Autodesk Inventor part; units mm, degrees
ref_plane "Plan de construction1" through (0, 10, 0) normal (0, 1, 0) x (-1, 0, 0)
ref_plane "YZ Plane" through (0, 0, 0) normal (1, 0, 0) x (0, 1, 0)
ref_plane "XY Plane" through (0, 0, 0) normal (0, 0, 1) x (1, 0, 0)
sketch "Esquisse1" plane through (0, 0, 0) normal (0, 0, 1) x (1, 0, 0)
  line L0 (0, 0) -> (0, 38)
  line L1 (0, 38) -> (30, 38)
  line L2 (30, 38) -> (30, 35.5)
  line L3 (30, 35.5) -> (0, 35.5)
  line L4 (0, 0) -> (0, 10)
  line L5 (0, 10) -> (18, 10)
  line L6 (18, 10) -> (18, 0)
  line L7 (18, 0) -> (0, 0)
  line L8 (-6, 0) -> (36, 0)
  dimension "d0" = 38
  dimension "d1" = 30
  dimension "d2" = 2.5
  dimension "d3" = 10
  dimension "d4" = 18
revolve "Révolution1" add sketch "Esquisse1" angle 360 about axis through (-10, 0, 0) along (1, 0, 0)
ref_plane "Plan de construction1" through (0, 10, 0) normal (0, 1, 0) x (-1, 0, 0)
sketch "Esquisse2" plane through (0, 10, 0) normal (0, 1, 0) x (-1, 0, 0)
  line L0 (0, 0) -> (0, 1)
  line L1 (0, 38) -> (0, -38)
  line L2 (0, 1) -> (-18, 1)
  line L3 (-18, 1) -> (-18, -1)
  line L4 (-18, -1) -> (0, -1)
  line L5 (0, 0) -> (0, -1)
  dimension "d7" = 1
  dimension "d8" = 18
  dimension "d9" = 2
  dimension "d10" = 90
extrude "Extrusion1" add sketch "Esquisse2" along normal up to surface
sketch "Esquisse3" plane through (30, 0, 0) normal (1, 0, 0) x (0, 0, -1)
  circle A0 centre (0, 0) radius 38
  circle A1 centre (0, 0) radius 38
  line L0 (0, 38) -> (0, 40)
  line L1 (0, 40) -> (0.5, 40)
  line L2 (0.5, 40) -> (0.5, 37.9967)
  line L3 (0, 40) -> (-0.5, 40)
  line L4 (-0.5, 40) -> (-0.5, 37.9967)
  dimension "d13" = 2
  dimension "d14" = 0.5
  dimension "d15" = 0.5
extrude "Extrusion2" add sketch "Esquisse3" against normal blind 30 contours A0 L0 L1 L2 | L4 L3 L0 A0
pattern_circular "Réseau circulaire1" count 10 over 360 about axis through (9, 0, 0) along (1, 0, 0) of "Extrusion1"
pattern_circular "Réseau circulaire2" count 40 over 360 about axis through (9, 0, 0) along (1, 0, 0) of "Extrusion2"
sketch "Esquisse4" plane through (0, 0, 0) normal (-1, 0, 0) x (0, 0, 1)
  circle A0 centre (0, 0) radius 2.85
  circle A1 centre (0, 0) radius 2.65
  line L0 (2.65, 0) -> (-2, 0)
  line L1 (-2, 0) -> (-2, 1.7385)
  line L2 (-2, 0) -> (-2, -1.7385)
  point P0 (-1.816, -1.3284)
  point P1 (-1.816, 1.3284)
  dimension "d24" = 5.7
  dimension "d25" = 5.3
  dimension "d26" = 4.65
extrude "Extrusion3" cut sketch "Esquisse4" against normal blind 25 contours L0 L1 A1 | A1 L2 L0
sketch "Esquisse7" plane through (0, 0, 0) normal (-1, 0, 0) x (0, 0, 1)
  circle A0 centre (0, 0) radius 2.55
  dimension "d30" = 5.1
extrude "Extrusion4" cut sketch "Esquisse7" against normal blind 7
sketch "Esquisse8" plane through (0, 0, 0) normal (-1, 0, 0) x (0, 0, 1)
  arc A0 (-2, 1.5819) -> (-2, -1.5819) centre (0, 0) ccw
  circle A1 centre (0, 0) radius 35.5
  line L0 (-2, 1.5819) -> (-2, -1.5819)
  arc A2 (-2, 1.5819) -> (-2, -1.5819) centre (0, 0) ccw
extrude "Extrusion5" cut sketch "Esquisse8" against normal blind 4 contours L0 A0 | A1
sketch "Esquisse9" plane through (18, 0, 0) normal (1, 0, 0) x (0, 0, -1)
  arc A0 (2, -1.5819) -> (2, 1.5819) centre (0, 0) ccw
  circle A1 centre (0, 0) radius 7.0446
  circle A2 centre (0, 0) radius 44.6529
extrude "Extrusion6" cut sketch "Esquisse9" along normal through all both and the other way through all
properties part number "Roue test"
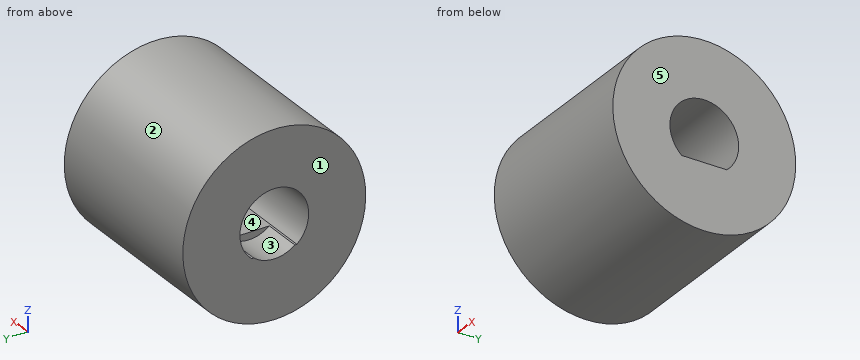
Could you check a few things on this model? Use its own coordinates, in mm. Face numbers are marked on the shaded views. A direction names the side the tool comes from. Give positions to 0.01 mm unless a question says otherwise; leave off trailing zeros. Write each loop counter-clockwise with the first axis right and the second up, starting at its lowest first coordinate (ties: lowest second). Pieces come first, ordered by that corner, then holes. Notation, with made-up numbers: (55.5, -33.75) -> (61.5, -33.75) arc R15 cw to (61.5, -8.75) -> close; hole circle Ø4 at (50, -19). An arc over 180 degrees is marked (long way). Write each question's results on one line, items separated by ' | '. Start each with the question number.
Q1. Suppose I cut it at A-A, the plane z = 0. List the corners of the cut face in (x, y) for me, and give its area (3 significant figures).
Q2. We'd pull the mould along Y, two halves only. Please class the marked faces 1, 2 and 3: +Y half, -Y half, draft (parallel to the pull), parting line (faces both ways), or undercut.
Q3. Which directions (+Z, -Z, +X, -X, +Y, -Y) give clear straight access to the entire face, cutting with the end or side of a thin tool? Please do the marked faces 4 and 5.
Q4. Suppose I cut it at D-D, the plane z = 2.25. List the corners of the cut face in (x, y) for me, and give its area (3 significant figures).
Q5. Suppose I cut it at C-C, the plane x = 8.5. List the corners of the cut face in (y, z) for me.
Q6. I'm going to push flat-ended pins straight in: pin 1 Ø4 at (x, y) = (14, 4.5) entering from +Z; pin 2 Ø3 at (x, z) = (15.5, 4) entering from -Y; pin 3 Ø2 at (x, y) = (8.5, -2) entering from +Z. Where does each tip first touch, or does it pass through?
Q7. I need wall thicknesses on probe 1 along Y at (x, z) = (10.5, 0); probe 2 along Z at (x, y) = (13.5, 1.75); probe 3 along Z at (x, y) = (8.25, 2). Which ranges of each line are inside material? Lowest first, please.
Q8. Suppose I cut it at B-B, the plane y = -0.5. List the corners of the cut face in (x, z) for me.
Outcome:
1) outline: (4, -7.04) -> (18, -7.04) -> (18, -2.65) -> (4, -2.65) -> close; (4, 2.65) -> (18, 2.65) -> (18, 7.04) -> (4, 7.04) -> close | area: 123 mm2
2) face 1: draft | face 2: parting line | face 3: undercut
3) face 4: +X, -X | face 5: +Z, -Z, +X, +Y, -Y
4) outline: (4, -6.68) -> (18, -6.68) -> (18, -1.4) -> (4, -1.4) -> close; (4, 1.4) -> (18, 1.4) -> (18, 6.68) -> (4, 6.68) -> close | area: 148 mm2
5) outline: circle Ø14.09 at (0, 0); hole (-1.74, -2) -> (1.74, -2) arc R2.65 ccw (long way) to start
6) pin 1: z = 6.59 | pin 2: y = -6.59 | pin 3: z = 6.97
7) probe 1: -7.04 to -2.65, 2.65 to 7.04 | probe 2: -6.82 to -1.99, 1.99 to 6.82 | probe 3: -6.75 to -1.74, 1.74 to 6.75
8) outline: (4, -7.03) -> (18, -7.03) -> (18, -2) -> (7, -2) -> (7, -2.5) -> (4, -2.5) -> close; (4, 2.6) -> (18, 2.6) -> (18, 7.03) -> (4, 7.03) -> close
